from build123d import *

# Parameters (mm, degrees)
SKETCH1_R            = 11
SKETCH1_R_2          = 7.5
EXTRUDE_THIN1_DEPTH  = 10
BOSS_EXTRUDE2_DEPTH  = 10
SKETCH6_W            = 10
SKETCH6_H            = 5
BOSS_EXTRUDE3_DEPTH  = 10
SKETCH8_W            = 10
SKETCH8_H            = 5
BOSS_EXTRUDE4_DEPTH  = 10
SKETCH9_W            = 42
SKETCH9_H            = 5
BOSS_EXTRUDE5_DEPTH  = 54
LPATTERN3_COUNT      = 2
LPATTERN3_PITCH      = 54
SKETCH15_R           = 11
BOSS_EXTRUDE6_DEPTH  = 10
SKETCH17_R           = 7.5
CUT_EXTRUDE1_DEPTH   = 10
SKETCH19_W           = 38
SKETCH19_H           = 38
CUT_EXTRUDE3_DEPTH   = 3
SKETCH25_W           = 29
SKETCH25_H           = 29
CUT_EXTRUDE4_DEPTH   = 2
SKETCH26_R           = 1.00264766
CUT_EXTRUDE5_DEPTH   = 3
LPATTERN4_COUNT      = 2
LPATTERN4_PITCH      = 36
LPATTERN4_COUNT_DIR2 = 2
LPATTERN4_PITCH_DIR2 = 41


with BuildPart() as part:
    # Sketch1 → Extrude-Thin1 (new body)
    with BuildSketch(Plane(origin=(0, 0, 0), x_dir=(0, 0, -1), z_dir=(1, 0, 0))):
        Circle(SKETCH1_R)
        Circle(SKETCH1_R_2, mode=Mode.SUBTRACT)
    extrude(amount=EXTRUDE_THIN1_DEPTH)

    # Sketch3 → Boss-Extrude2 (add)
    with BuildSketch(Plane(origin=(0, 0, 0), x_dir=(0, 0, -1), z_dir=(1, 0, 0))):
        with BuildLine():
            Line((-11, 0), (-11, 30))
            Line((-11, 30), (11, 30))
            Line((11, 30), (11, 0))
            ThreePointArc((11, 0), (0, 11), (-11, 0))
        make_face()
    boss_extrude2 = extrude(amount=BOSS_EXTRUDE2_DEPTH)

    # Sketch6 → Boss-Extrude3 (add)
    with BuildSketch(Plane.XY.offset(11)):
        with Locations((5, 27.5)):
            Rectangle(SKETCH6_W, SKETCH6_H)
    extrude(amount=BOSS_EXTRUDE3_DEPTH)

    # Sketch8 → Boss-Extrude4 (add)
    with BuildSketch(Plane(origin=(0, 0, -11), x_dir=(-1, 0, 0), z_dir=(0, 0, -1))):
        with Locations((-5, 27.5)):
            Rectangle(SKETCH8_W, SKETCH8_H)
    extrude(amount=BOSS_EXTRUDE4_DEPTH)

    # Sketch9 → Boss-Extrude5 (add)
    with BuildSketch(Plane.ZY):
        with Locations((0, 27.5)):
            Rectangle(SKETCH9_W, SKETCH9_H)
    extrude(amount=BOSS_EXTRUDE5_DEPTH)

    # LPattern3: Boss-Extrude2 ×2
    with Locations(*[(-i * LPATTERN3_PITCH, 0, 0) for i in range(1, LPATTERN3_COUNT)]):
        add(boss_extrude2)

    # Sketch15 → Boss-Extrude6 (add)
    with BuildSketch(Plane.ZY.offset(54)):
        Circle(SKETCH15_R)
    extrude(amount=-BOSS_EXTRUDE6_DEPTH)

    # Sketch17 → Cut-Extrude1 (cut)
    with BuildSketch(Plane.ZY.offset(54)):
        with Locations(Location((0, 0, 0), (0, 0, 180))):
            Circle(SKETCH17_R)
    extrude(amount=-CUT_EXTRUDE1_DEPTH, mode=Mode.SUBTRACT)

    # Sketch19 → Cut-Extrude3 (cut)
    with BuildSketch(Plane(origin=(0, 30, 0), x_dir=(1, 0, 0), z_dir=(0, 1, 0))):
        with Locations((-22, 0)):
            Rectangle(SKETCH19_W, SKETCH19_H)
    extrude(amount=-CUT_EXTRUDE3_DEPTH, mode=Mode.SUBTRACT)

    # Sketch25 → Cut-Extrude4 (cut)
    with BuildSketch(Plane(origin=(0, 27, 0), x_dir=(1, 0, 0), z_dir=(0, 1, 0))):
        with Locations((-22.144950272, -0.049169749)):
            Rectangle(SKETCH25_W, SKETCH25_H)
    extrude(amount=-CUT_EXTRUDE4_DEPTH, mode=Mode.SUBTRACT)

    # Sketch26 → Cut-Extrude5 (cut)
    with BuildSketch(Plane(origin=(0, 30, 0), x_dir=(1, 0, 0), z_dir=(0, 1, 0))):
        with Locations(Location((-1.5, 17.99735234, 0), (0, 0, 270))):
            Circle(SKETCH26_R)
    cut_extrude5 = extrude(amount=-CUT_EXTRUDE5_DEPTH, mode=Mode.SUBTRACT)

    # LPattern4: Cut-Extrude5 2 × 2
    with Locations(*[(-j * LPATTERN4_PITCH_DIR2, 0, i * LPATTERN4_PITCH) for i in range(LPATTERN4_COUNT) for j in range(LPATTERN4_COUNT_DIR2) if (i, j) != (0, 0)]):
        add(cut_extrude5, mode=Mode.SUBTRACT)


solid = part.part
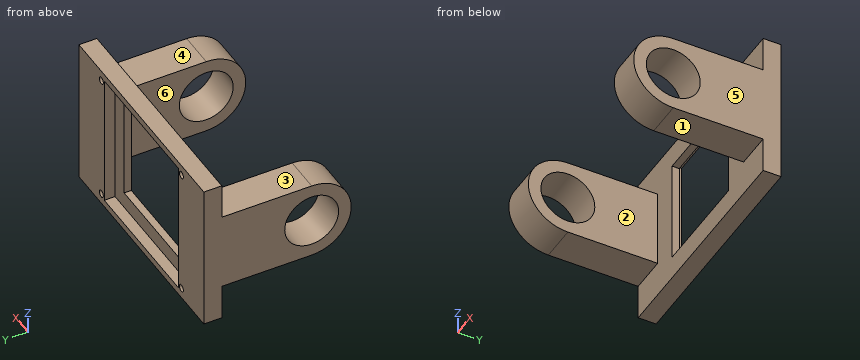
Here's how the part is built. I have some questions about the finished solid (model axes, mm). Face numbers are marked on the shaded views. A direction names the side the tool comes from. Coordinates: 2 decimals unless noted, no trailing zeros. Loops run counter-clockwise (first coordinate to the right, second up) from the corner with the lowest first, then second, coordinate; pieces in that order, holes last.
1. I need wall thicknesses on L1, parallel to Z at x = -35, y = 26.5; L2, parallel to Y at x = 3.75, z = 0; L3, parallel to X at y = 17, z = -3. Which ranges of each line are inside material? Lowest first, please.
2. Imagine slicing it at C-C, the plane y = 11. Please give me the cut outline in (x, z), and give its area (3 significant figures).
3. If we mould it in two halves opening along X, with no side actions, what happens to the marked faces 4, 5 and 6? For each: pulls with the +X half, pulls with the -X half, needs draft (parallel to the pull), parting line crosses it, or undercut.
4. For P1, Ø11.5, axis at x = -28, z = -7.5, coming from the +Y side; P2, Ø3, axis at x = -1, y = -2.5, coming from the +Z side; P3, Ø3, axis at x = 4, y = 6.5, coming from the -Z side; P4, Ø5, axis at x = -50, y = 13.5, coming from the +Z side, each with a flat end and sliding along its axis, tell me the tip position at first contact or that it passes through.
5. Imagine slicing it at B-B, the plane z = 13. Please give me the cut outline in (x, y), and give its area (3 significant figures).
6. Imagine slicing it at D-D, the plane z = 0. Please give me the cut outline in (x, y).
7. For the marked faces 1, 2 and 3, which set-ups out of +Z, -Z, +X, -X, +Y, -Y let a thin tool reach every point of the face, with its end or its side?
8. Imagine slicing it at A-A, the plane x = -28. Please give me the cut outline in (y, z), and give its area (3 significant figures).
Taken from the geometry:
1. L1: z = -21 to -14.45, 14.55 to 21
1. L2: y = -11 to -7.5, 7.5 to 30
1. L3: x = -54 to -44, 0 to 10
2. outline: (-54, -11) - (-44, -11) - (-44, 11) - (-54, 11) - close; (0, -11) - (10, -11) - (10, 11) - (0, 11) - close
2. area: 440 mm2
3. face 4: needs draft
3. face 5: pulls with the +X half
3. face 6: undercut
4. P1: passes through
4. P2: stops at z = 10.91
4. P3: stops at z = -11
4. P4: stops at z = 11
5. outline: (-54, 25) - (-36.64, 25) - (-36.64, 27) - (-41, 27) - (-41, 30) - (-54, 30) - close; (-7.64, 25) - (10, 25) - (10, 30) - (-3, 30) - (-3, 27) - (-7.64, 27) - close
5. area: 148 mm2
6. outline: (-54, -11) - (-44, -11) - (-44, -7.5) - (-54, -7.5) - close; (-54, 7.5) - (-44, 7.5) - (-44, 25) - (-36.64, 25) - (-36.64, 27) - (-41, 27) - (-41, 30) - (-54, 30) - close; (-7.64, 25) - (0, 25) - (0, 7.5) - (10, 7.5) - (10, 30) - (-3, 30) - (-3, 27) - (-7.64, 27) - close; (0, -11) - (10, -11) - (10, -7.5) - (0, -7.5) - close
7. face 1: -Z, +X, -X, -Y
7. face 2: +Z, -Z, -Y
7. face 3: +Z, +X, -X, -Y
8. outline: (25, -21) - (30, -21) - (30, -19) - (27, -19) - (27, -14.45) - (25, -14.45) - close; (25, 14.55) - (27, 14.55) - (27, 19) - (30, 19) - (30, 21) - (25, 21) - close
8. area: 38.0 mm2
